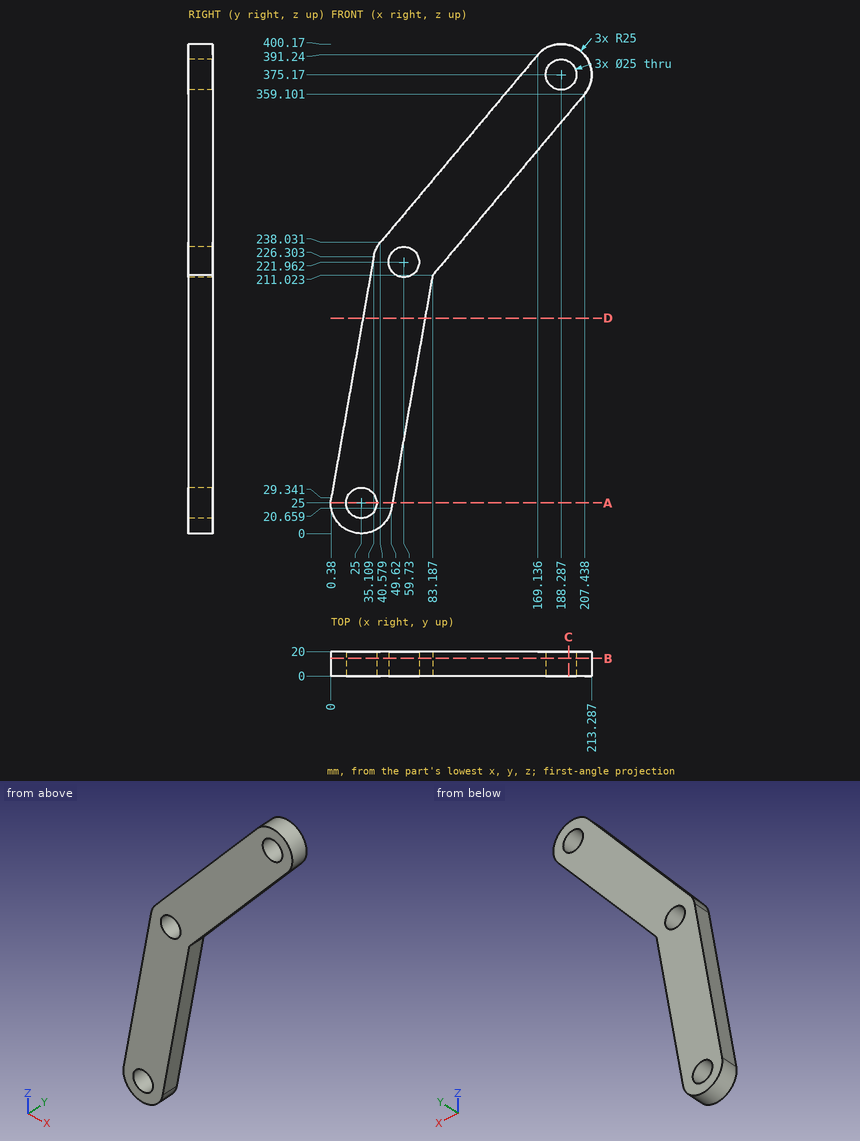
Here's the drawing with two shaded views (mm, measured from the low corner). I have some questions. Coordinates: 2 decimals unless noted, no trailing zeros. Write each loop counter-clockwise with the first axis right and the second up, starting at its lowest first coordinate (ties: lowest second). Pieces come first, ordered by that corner, then holes. Notation, with made-up numbers: (80.5, 0.25) -> (137.5, 0.25) arc R22 cw to (137.5, 39.25) -> close; hole circle Ø10 at (0, -40). An arc over 180 degrees is marked (long way). One line per question, with ' | ' between items. Start each with the question number.
1. If we section it at A-A (z = 25): Please give me the cut outline in (x, y) (1 decimal), and give its area (3 significant figures).
2. Please list where these lines run through material, in increasing order: line 1 along Z through (x, y) = (197, 9.25) (1 decimal); line 2 along Z through (x, y) = (178.5, 8.75) (1 decimal); line 3 along X through (y, z) = (5.5, 25) (1 decimal).
3. If we section it at C-C (x = 194.5): Please give me the cut outline in (y, z).
4. If we section it at B-B (y = 14.5): Please give me the cut outline in (x, z) (1 decimal), and give its area (3 significant figures).
5. If we section it at D-D (z = 176): Please give me the cut outline in (x, y).
6. Will these pins go through, and if not, where does the flat tip stop? P1, Ø1, axis at y = 2, z = 338.5, coming from the -X side; P2, Ø2, axis at x = 45.5, y = 13.5, coming from the -Z side (1 decimal); P3, Ø10, axis at x = 150, y = 10.5, coming from the -Z side.
Return value:
1) outline: (0, 0) -> (12.5, 0) -> (12.5, 20) -> (0, 20) -> close; (37.5, 0) -> (50.4, 0) -> (50.4, 20) -> (37.5, 20) -> close | area: 508 mm²
2) line 1: z = 346.7 to 366.2, 384.1 to 398.6 | line 2: z = 324.6 to 367.4, 382.9 to 398.2 | line 3: x = 0 to 12.5, 37.5 to 50.4
3) outline: (0, 343.68) -> (20, 343.68) -> (20, 364.32) -> (0, 364.32) -> close; (0, 386.02) -> (20, 386.02) -> (20, 399.39) -> (0, 399.39) -> close
4) outline: (0.4, 29.3) arc R25 ccw to (49.6, 20.7) -> (83.2, 211) -> (207.4, 359.1) arc R25 ccw to (169.1, 391.2) -> (40.6, 238) arc R25 ccw to (35.1, 226.3) -> close; hole circle Ø25 at (25, 25); hole circle Ø25 at (59.7, 222); hole circle Ø25 at (188.3, 375.2) | area: 20,500 mm²
5) outline: (26.24, 0) -> (77.01, 0) -> (77.01, 20) -> (26.24, 20) -> close
6) P1: stops at x = 124.46 | P2: stops at z = 9.4 | P3: stops at z = 284.69
